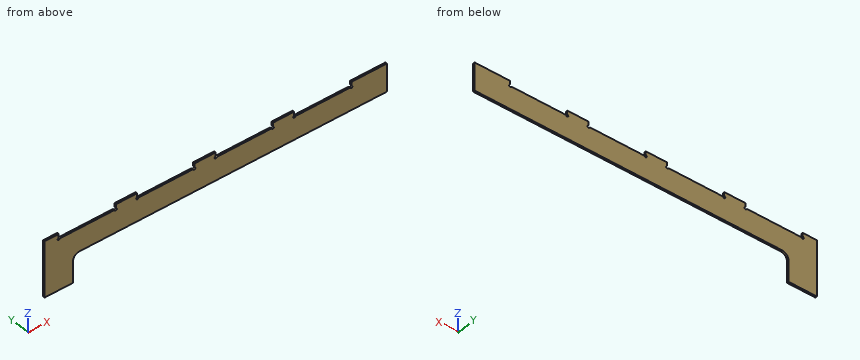
from build123d import *

# Parameters (mm, degrees)
F1_DEPTH = 6.35
F3_DEPTH = 6.351
F4_R     = 5.08
F5_R     = 23.301989


with BuildPart() as f1:
    # F0 (on Front) → F1 (new body)
    with BuildSketch(Plane.XZ):
        Polygon((0, 203.2), (0, 0), (101.6, 0), (101.6, 101.6), (1219.2, 101.6), (1219.2, 203.2), align=None)
    extrude(amount=F1_DEPTH)

    # F2 (on face) → F3 (cut, through all)
    with BuildSketch(Plane.XZ.offset(6.35)):
        with BuildLine():
            Line((254, 184.9882), (250.19, 184.9882))
            ThreePointArc((250.19, 184.9882), (256.694077, 182.294123), (254, 188.7982))
            Line((254, 188.7982), (254, 184.9882))
        make_face()
        with BuildLine():
            Line((50.8, 184.9882), (50.8, 188.7982))
            ThreePointArc((50.8, 188.7982), (48.105923, 182.294123), (54.61, 184.9882))
            Line((54.61, 184.9882), (50.8, 184.9882))
        make_face()
        with BuildLine():
            Line((533.4, 184.9882), (529.59, 184.9882))
            ThreePointArc((529.59, 184.9882), (536.094077, 182.294123), (533.4, 188.7982))
            Line((533.4, 188.7982), (533.4, 184.9882))
        make_face()
        with BuildLine():
            Line((330.2, 184.9882), (330.2, 188.7982))
            ThreePointArc((330.2, 188.7982), (327.505923, 182.294123), (334.01, 184.9882))
            Line((334.01, 184.9882), (330.2, 184.9882))
        make_face()
        with BuildLine():
            Line((812.8, 184.9882), (808.99, 184.9882))
            ThreePointArc((808.99, 184.9882), (815.494077, 182.294123), (812.8, 188.7982))
            Line((812.8, 188.7982), (812.8, 184.9882))
        make_face()
        with BuildLine():
            Line((609.6, 184.9882), (609.6, 188.7982))
            ThreePointArc((609.6, 188.7982), (606.905923, 182.294123), (613.41, 184.9882))
            Line((613.41, 184.9882), (609.6, 184.9882))
        make_face()
        with BuildLine():
            Line((1092.2, 184.9882), (1088.39, 184.9882))
            ThreePointArc((1088.39, 184.9882), (1094.894077, 182.294123), (1092.2, 188.7982))
            Line((1092.2, 188.7982), (1092.2, 184.9882))
        make_face()
        with BuildLine():
            Line((889, 184.9882), (889, 188.7982))
            ThreePointArc((889, 188.7982), (886.305923, 182.294123), (892.81, 184.9882))
            Line((892.81, 184.9882), (889, 184.9882))
        make_face()
        Polygon((254, 203.2), (50.8, 203.2), (50.8, 188.7982), (50.8, 184.9882), (54.61, 184.9882), (152.4, 184.9882), (250.19, 184.9882), (254, 184.9882), (254, 188.7982), align=None)
        Polygon((533.4, 203.2), (330.2, 203.2), (330.2, 188.7982), (330.2, 184.9882), (334.01, 184.9882), (431.8, 184.9882), (529.59, 184.9882), (533.4, 184.9882), (533.4, 188.7982), align=None)
        Polygon((812.8, 203.2), (609.6, 203.2), (609.6, 188.7982), (609.6, 184.9882), (613.41, 184.9882), (711.2, 184.9882), (808.99, 184.9882), (812.8, 184.9882), (812.8, 188.7982), align=None)
        Polygon((1092.2, 203.2), (889, 203.2), (889, 188.7982), (889, 184.9882), (892.81, 184.9882), (990.6, 184.9882), (1088.39, 184.9882), (1092.2, 184.9882), (1092.2, 188.7982), align=None)
    extrude(amount=-F3_DEPTH, mode=Mode.SUBTRACT)

    # F4
    f4_edges = [f1.edges().sort_by_distance(p)[0] for p in [
        (334.01, -3.175, 184.9882),
        (330.2, -3.175, 188.7982),
        (529.59, -3.175, 184.9882),
        (533.4, -3.175, 188.7982),
        (54.61, -3.175, 184.9882),
        (50.8, -3.175, 188.7982),
        (250.19, -3.175, 184.9882),
        (254, -3.175, 188.7982),
        (1092.2, -3.175, 188.7982),
        (1088.39, -3.175, 184.9882),
        (812.8, -3.175, 188.7982),
        (808.99, -3.175, 184.9882),
        (609.6, -3.175, 188.7982),
        (613.41, -3.175, 184.9882),
        (889, -3.175, 188.7982),
        (892.81, -3.175, 184.9882),
    ]]
    fillet(f4_edges, radius=F4_R)

    # F5
    f5_edges = [f1.edges().sort_by_distance(p)[0] for p in [
        (101.6, -3.175, 101.6),
    ]]
    fillet(f5_edges, radius=F5_R)


solid = f1.part
Source: CAD feature listing. Evaluate the final solid. Frame: model axes, mm. Round coordinates to 2 decimals unless told otherwise and drop trailing zeros. Write each loop counter-clockwise with the first axis right and the second up, starting at its lowest first coordinate (ties: lowest second). Pieces come first, ordered by that corner, then holes. Notation, with made-up numbers: (-24, 19) - (28, 19) arc R24 cw to (28, 37) - close; hole circle Ø7 at (-25, 37.25). An arc over 180 degrees is marked (long way). Use CSV: the item, a comma, the result in double quotes. Start each with the question number.
(1) First-contact query: pin 1 Ø3 at (x, y) = (402, -3.5) entering from +Z. Flat tip, straight axial feed; report the tip coordinate or a pass-through.
(2) Cut plane A-A, the plane x = 1134. Return loops of the section in (y, z).
(3) Material intervals for probe 1 along X at (y, z) = (-1.25, 192); probe 2 along X at (y, z) = (-1, 29.5); probe 3 along Z at (x, y) = (448.5, -6), sorted ascending. Write a range as [from, to].
(4) Cut plane B-B, the plane z = 89.5. Return loops of the section in (x, y).
Geometry says:
1,pin 1,"z = 184.99"
2,outline,"(-6.35, 101.6) - (0, 101.6) - (0, 203.2) - (-6.35, 203.2) - close"
3,probe 1,"[0, 50.79], [254.01, 330.19], [533.41, 609.59], [812.81, 888.99], [1092.21, 1219.2]"
3,probe 2,"[0, 101.6]"
3,probe 3,"[101.6, 184.99]"
4,outline,"(0, -6.35) - (104.47, -6.35) - (104.47, 0) - (0, 0) - close"
